Work out the finished part from the listing and answer in its coordinate system (mm). A direction names the side the tool comes from. Round coordinates to 2 decimals unless told otherwise and drop trailing zeros. Write each loop counter-clockwise with the first axis right and the second up, starting at its lowest first coordinate (ties: lowest second). Pieces come first, ordered by that corner, then holes. Notation, with made-up numbers: (50, 75.25) - (104, 75.25) arc R16 ccw to (104, 95.25) - close; hole circle Ø8 at (66, 86). An arc over 180 degrees is marked (long way). Answer as a JSON object with one key per item and string values.
```python
from build123d import *

# Parameters (mm, degrees)
F0_R     = 15.286331743
F0_R_2   = 12
F1_DEPTH = 68.326
F2_R     = 15.286331743
F3_DEPTH = 25.4
F3_TAPER = 35
F4_R     = 63.5


with BuildPart() as f1:
    # F0 (on Top) → F1 (new body)
    with BuildSketch(Plane.XY):
        Circle(F0_R)
        Circle(F0_R_2, mode=Mode.SUBTRACT)
    extrude(amount=F1_DEPTH)

    # F2 (on face) → F3 (join)
    with BuildSketch(Plane.XY.offset(68.326)):
        Circle(F2_R)
    extrude(amount=F3_DEPTH, taper=F3_TAPER)

    # F4
    f4_edges = [f1.edges().sort_by_distance(p)[0] for p in [
        (-15.286332, 0, 68.326),
    ]]
    fillet(f4_edges, radius=F4_R)


solid = f1.part
```
Item 1: For faces 1 (the conical face through (1.385, 0.436, 88.083)), 2 (the cylindrical face through (-11.99, 0.53, 33.68)), determine the directions among +Z, -Z, +X, -X, +Y, -Y from which every point of the face is accessible in a straight line to the end or side of a thin tool.
Results found:
{"face 1": "+Z", "face 2": "-Z"}
Item 2: Each of these flat-tipped pins is pushed along its axis until it touches: P1, Ø1, axis at y = 2, z = 75, coming from the +X side; P2, Ø3, axis at y = 0, z = 77.5, coming from the -X side; P3, Ø2, axis at x = 8.5, y = 2.5, coming from the +Z side; P4, Ø12, axis at x = -4, y = -5.5, coming from the -Z side. Where does it stop, or does it pass through?
Results found:
{"P1": "x = 9.44", "P2": "x = -8.93", "P3": "z = 78.1", "P4": "z = 0"}
Item 3: A cutting plane is placed at A-A (z = 19). Write down the section's boundary in (x, y).
Results found:
{"outline": "circle Ø30.57 at (0, 0); hole circle Ø24 at (0, 0)"}
Item 4: Determine the mould class of faces 3 (the cylindrical face through (-3.314, -14.923, 23.814)), 4 (the flat face through (7, -10, 0)), 5 (the flat face through (0, 0, 68.326)) for opening direction Y: pulls with the +Y half, pulls with the -Y half, needs draft (parallel to the pull), parting line crosses it, or undercut.
Results found:
{"face 3": "parting line crosses it", "face 4": "needs draft", "face 5": "undercut"}
Item 5: Consider line 1 along Y through (x, z) = (0, 27); line 2 along Y through (x, z) = (5.5, 4); line 3 along X through (y, z) = (-5, 46). Determine where each line is inside the solid, lowest interval first.
Results found:
{"line 1": "-15.29 to -12, 12 to 15.29", "line 2": "-14.26 to -10.67, 10.67 to 14.26", "line 3": "-14.45 to -10.91, 10.91 to 14.45"}
